from build123d import *

# Parameters (mm, degrees)
BOSS_EXTRUDE1_DEPTH        = 6.35
BOSS_EXTRUDE2_DEPTH        = 44.45
CUT_EXTRUDE2_DEPTH         = 1
CUT_EXTRUDE2_DEPTH_BACK    = 34.925
F_10_32_TAPPED_HOLE1_D     = 4.0386
F_10_32_TAPPED_HOLE1_DEPTH = 6.35
BOSS_EXTRUDE5_DEPTH        = 3.175
CIRPATTERN1_COUNT          = 2
CIRPATTERN1_ANGLE          = 47.375
FILLET1_R                  = 4.7625


with BuildPart() as part:
    # Sketch1 → Boss-Extrude1 (new body)
    with BuildSketch(Plane(origin=(0, 0, 0), x_dir=(1, 0, 0), z_dir=(0, 1, 0))):
        with BuildLine():
            Line((0, 146.558), (0, 165.608))
            ThreePointArc((0, 165.608), (-117.102539819, 117.102539819), (-165.608, 0))
            Line((-165.608, 0), (-146.558, 0))
            ThreePointArc((-146.558, 0), (-103.632155637, 103.632155637), (0, 146.558))
        make_face()
    extrude(amount=BOSS_EXTRUDE1_DEPTH)

    # Sketch4 → Boss-Extrude2 (add)
    with BuildSketch(Plane(origin=(0, 6.35, 0), x_dir=(1, 0, 0), z_dir=(0, 1, 0))):
        with BuildLine():
            Line((-149.733, 0), (-146.558, 0))
            ThreePointArc((-146.558, 0), (-103.632155637, 103.632155637), (0, 146.558))
            Line((0, 146.558), (0, 149.733))
            ThreePointArc((0, 149.733), (-105.877219667, 105.877219667), (-149.733, 0))
        make_face()
    extrude(amount=BOSS_EXTRUDE2_DEPTH)

    # Sketch5 → Cut-Extrude2 (cut, two sides)
    with BuildSketch(Plane(origin=(0, 50.8, 0), x_dir=(1, 0, 0), z_dir=(0, 1, 0))) as cut_extrude2_sk:
        with BuildLine():
            Line((-146.558, 0), (-149.733, 0))
            ThreePointArc((-149.733, 0), (-140.20067708, 52.57129859), (-112.817404434, 98.448994641))
            Line((-112.817404434, 98.448994641), (-110.567041393, 96.198631599))
            ThreePointArc((-110.567041393, 96.198631599), (-137.265676366, 51.355442319), (-146.558, 0))
        make_face()
    extrude(amount=CUT_EXTRUDE2_DEPTH, mode=Mode.SUBTRACT)
    extrude(cut_extrude2_sk.sketch, amount=-CUT_EXTRUDE2_DEPTH_BACK, mode=Mode.SUBTRACT)

    # #10-32 Tapped Hole1
    with Locations(Plane(origin=(0, 6.35, 0), x_dir=(1, 0, 0), z_dir=(0, 1, 0))):
        with Locations((-6.35, 157.542578595), (-87.858258413, 130.923309609), (-143.383000088, 65.58431105)):
            Hole(F_10_32_TAPPED_HOLE1_D / 2, depth=F_10_32_TAPPED_HOLE1_DEPTH)

    # Sketch9 → Boss-Extrude5 (add)
    with BuildSketch(Plane(origin=(0, 0, 0), x_dir=(0, 0, -1), z_dir=(1, 0, 0))):
        Polygon((149.733, 50.8), (165.608, 6.35), (146.558, 6.35), (146.558, 50.8), align=None)
    boss_extrude5 = extrude(amount=-BOSS_EXTRUDE5_DEPTH)

    # CirPattern1: Boss-Extrude5 ×2 about axis
    cirpattern1_axis = Axis((0, 0, 0), (0, 1, 0))
    for i in range(1, CIRPATTERN1_COUNT):
        add(boss_extrude5.rotate(cirpattern1_axis, i * CIRPATTERN1_ANGLE / (CIRPATTERN1_COUNT - 1)))

    # Fillet1
    fillet1_edges = [part.edges().sort_by_distance(p)[0] for p in [
        (-61.605387238, 6.35, -136.472515739),
        (-140.062228399, 6.35, -52.939054251),
    ]]
    fillet(fillet1_edges, radius=FILLET1_R)


solid = part.part
The listing builds one solid part. Answer for the finished solid, in the listing's coordinates (mm). A direction names the side the tool comes from. Give positions to 0.01 mm unless a question says otherwise; leave off trailing zeros. Order: outer loops, then holes, each group sorted by start corner. A loop starts at its lowest first (then second) coordinate and runs counter-clockwise, first axis right, second up. Notation, with made-up numbers: (66.5, 29) - (86.5, 29) arc R34 ccw to (86.5, 67) - close; hole circle Ø1 at (37, 29.5). An arc over 180 degrees is marked (long way). One line per item, written item: value. Start each with the question number.
1) The mould has two halves that part along X. Classify faces 4 (the face through (-115.633, 19.008, -102.108)), 5 (the face through (-89.7, 3.1, -130.1)), 6 (the face through (-85.38, 19.4, -119.12)), 7 (the face through (-148, 6.35, -55)): released by +X, released by -X, zero draft, split by the parting line, or undercut.
2) A cutting plane is placed at A-A on y = 20. Give the vertices of the cut face in (x, z) (3 decimals).
3) A tool of negligible diameter and unlimited length cuts with its end or side. For faces 1 (the face through (-139.97, 13.22, -53.18)), 2 (the face through (-113.5, 19.01, -104.46)), 3 (the face through (-3.175, 19, -154)), from which of +Z, -Z, +X, -X, +Y, -Y can it reach the whole face along a straight path? Write none if from no direction.
4) Given pin 1 Ø5 at (y, z) = (23.5, -130.5) entering from +X (3 decimals); pin 2 Ø1.5 at (x, y) = (-82, 16.5) entering from -Z; pin 3 Ø12.5 at (y, z) = (29, -160) entering from -X (3 decimals), each flat-ended and moving along its own axis, determine where each tip first touches the part or whether it passes through.
5) A cutting plane is placed at B-B on y = 30. Give the vertices of the cut face in (x, z) (3 decimals).
6) Find the intervals of material crossed by L1, parallel to X at y = 13.5, z = -101.5; L2, parallel to Y at x = -86, z = -141; L3, parallel to Z at x = -62.5, y = 31, in increasing order.
Answer sheet:
1. face 4: released by -X
1. face 5: undercut
1. face 6: released by +X
1. face 7: zero draft
2. outline: (-120.418, -106.512) - (-118.268, -108.848) - (-110.174, -101.399) arc R149.733 ccw to (-3.175, -149.699) - (-3.175, -160.733) - (0, -160.733) - (0, -146.558) arc R146.558 cw to (-110.567, -96.199) - (-112.817, -98.449) arc R149.733 ccw to (-112.299, -99.04) - close
3. face 1: -X, +Y
3. face 2: -Z, +Y
3. face 3: -Z, -X, +Y
4. pin 1: stops at x = -61.565
4. pin 2: stops at z = -125.77
4. pin 3: stops at x = -3.175
5. outline: (-117.79, -104.093) - (-115.64, -106.429) - (-110.174, -101.399) arc R149.733 ccw to (-3.175, -149.699) - (-3.175, -157.162) - (0, -157.162) - (0, -146.558) arc R146.558 cw to (-110.567, -96.199) - (-112.817, -98.449) arc R149.733 ccw to (-112.299, -99.04) - close
6. L1: x = -114.97 to -110.28, -110.08 to -105.72
6. L2: y = 0 to 6.35
6. L3: z = -136.07 to -132.56
